```python
from build123d import *

# Parameters (mm, degrees)
SKETCH1_R           = 3.5
BOSS_EXTRUDE1_DEPTH = 10
FILLET1_R           = 2
SKETCH4_R           = 4.5
CUT_EXTRUDE1_DEPTH  = 26
FILLET2_R           = 2


with BuildPart() as part:
    # Sketch1 → Boss-Extrude1 (new body)
    with BuildSketch(Plane.XY):
        with BuildLine():
            Line((57.741071939, 36.562090071), (56.204690111, 51.925908355))
            Line((56.204690111, 51.925908355), (46.264731801, 53.020087861))
            ThreePointArc((46.264731801, 53.020087861), (47.519621722, 46.969136515), (52.091231644, 42.811114916))
            Line((52.091231644, 42.811114916), (52.765885988, 36.064571476))
            Line((52.765885988, 36.064571476), (-12.906568566, 29.49732602))
            Line((-12.906568566, 29.49732602), (-12.011035094, 20.541991308))
            Line((-12.011035094, 20.541991308), (58.63660541, 27.606755359))
            Line((58.63660541, 27.606755359), (67.591940122, 28.50228883))
            Line((67.591940122, 28.50228883), (66.696406651, 37.457623542))
            Line((66.696406651, 37.457623542), (57.741071939, 36.562090071))
        make_face()
        with Locations((58.188838675, 32.084422715)):
            Circle(SKETCH1_R, mode=Mode.SUBTRACT)
    extrude(amount=BOSS_EXTRUDE1_DEPTH)

    # Fillet1
    fillet1_edges = [part.edges().sort_by_distance(p)[0] for p in [
        (56.204690111, 51.925908355, 5),
        (57.741071939, 36.562090071, 5),
        (66.696406651, 37.457623542, 5),
        (67.591940122, 28.50228883, 5),
        (52.765885988, 36.064571476, 5),
    ]]
    fillet(fillet1_edges, radius=FILLET1_R)

    # Sketch4 → Cut-Extrude1 (cut)
    with BuildSketch(Plane(origin=(0, 0, 0), x_dir=(1, 0, 0), z_dir=(0, 1, 0))):
        with Locations(Location((4.295066604, -5, 0), (0, 0, 180))):
            Circle(SKETCH4_R)
    extrude(amount=CUT_EXTRUDE1_DEPTH, mode=Mode.SUBTRACT)

    # Fillet2
    fillet2_edges = [part.edges().sort_by_distance(p)[0] for p in [
        (-12.011035094, 20.541991308, 5),
        (-12.906568566, 29.49732602, 5),
    ]]
    fillet(fillet2_edges, radius=FILLET2_R)


solid = part.part
```
Model file for the job. Use its own axes, mm. A direction names the side the tool comes from. Coordinates: 2 decimals unless noted, no trailing zeros. Order: outer loops, then holes, each group sorted by start corner. A loop starts at its lowest first (then second) coordinate and runs counter-clockwise, first axis right, second up. Notation, with made-up numbers: (-9.5, 46) -> (16.5, 46) arc R29 cw to (16.5, 72) -> close; hole circle Ø10 at (-12, 29). An arc over 180 degrees is marked (long way). Answer as a JSON object with one key per item and string values. Group by question number.
1) Which spindle directions (+Z, -Z, +X, -X, +Y, -Y) get a long thin tool onto all of the face, cutting with end or side? Do faces 1 (the face through (52.326, 40.466, 4.93)), 2 (the face through (62.254, 37.013, 4.93)), 3 (the face through (56.962, 44.351, 4.93)), 4 (the face through (4, 26, 5)). Say none if no direction does.
2) Flat gauge pins, fed straight in: pin 1 (4.5 mm diameter, centred on x = 6, z = 6, fed in from -Y); pin 2 (3 mm diameter, centred on x = 35, z = 4, fed in from -Y); pin 3 (2 mm diameter, centred on x = 32, y = 24, fed in from -Z); pin 4 (4 mm diameter, centred on y = 42.5, z = 7, fed in from +X). Where does each tip first touch, or does it go through?
3) Cut at B-B, the plane x = 48. Write the cut outline in (y, z).
4) Pull direction Z, two halves, no side cores. Call faces 5 (the face through (52.14, 36.61, 5.07)), 6 (the face through (30, 30, 10)), 7 (the face through (0.138, 24.307, 3.276)): +Z half, -Z half, draft (parallel to the pull), parting line (faces both ways), or undercut.
5) Drill centre lines: L1, parallel to Z at x = 3, y = 23; L2, parallel to Y at x = 8.5, z = 2.5; L3, parallel to X at y = 29, z = 4.5. Where is each one in solid material? Low to high.
6) Cut at A-A, the plane z = 6.5. Write the cut outline in (x, y).
7) Cut at D-D, the plane y = 46.5. Write the cut outline in (x, z), then the cut area to 3 significant figures.
8) Cut at C-C, the plane z = 1.25. Write the cut outline in (x, y).
Check values:
{
 "1": {"face 1": "+Z, -Z, -X", "face 2": "+Z, -Z, +Y", "face 3": "+Z, -Z, +X, +Y", "face 4": "-Y"},
 "2": {"pin 1": "stops at y = 26", "pin 2": "stops at y = 25.09", "pin 3": "stops at z = 0", "pin 4": "stops at x = 57.35"},
 "3": {"outline": "(26.54, 0) -> (35.59, 0) -> (35.59, 10) -> (26.54, 10) -> close; (46.21, 0) -> (52.83, 0) -> (52.83, 10) -> (46.21, 10) -> close"},
 "4": {"face 5": "draft", "face 6": "+Z half", "face 7": "undercut"},
 "5": {"L1": "z = 0 to 0.69, 9.31 to 10", "L2": "y = 22.59 to 31.64", "L3": "x = -12.24 to 56.53, 59.84 to 66.93"},
 "6": {"outline": "(-12.71, 27.51) -> (-12.21, 22.53) arc R2 ccw to (-10.02, 20.74) -> (0.05, 21.75) -> (0.05, 26) -> (8.54, 26) -> (8.54, 22.6) -> (65.6, 28.3) arc R2 ccw to (67.39, 30.49) -> (66.9, 35.47) arc R2 ccw to (64.71, 37.26) -> (59.73, 36.76) arc R2 cw to (57.54, 38.55) -> (56.37, 50.31) arc R2 ccw to (54.59, 52.1) -> (46.26, 53.02) arc R10 ccw to (52.09, 42.81) -> (52.57, 38.05) arc R2 cw to (50.78, 35.87) -> (-10.92, 29.7) arc R2 ccw to start; hole circle Ø7 at (58.19, 32.08)"},
 "7": {"outline": "(47.8, 0) -> (56.75, 0) -> (56.75, 10) -> (47.8, 10) -> close", "area": "89.4 mm²"},
 "8": {"outline": "(-12.71, 27.51) -> (-12.21, 22.53) arc R2 ccw to (-10.02, 20.74) -> (1.81, 21.92) -> (1.81, 26) -> (6.78, 26) -> (6.78, 22.42) -> (65.6, 28.3) arc R2 ccw to (67.39, 30.49) -> (66.9, 35.47) arc R2 ccw to (64.71, 37.26) -> (59.73, 36.76) arc R2 cw to (57.54, 38.55) -> (56.37, 50.31) arc R2 ccw to (54.59, 52.1) -> (46.26, 53.02) arc R10 ccw to (52.09, 42.81) -> (52.57, 38.05) arc R2 cw to (50.78, 35.87) -> (-10.92, 29.7) arc R2 ccw to start; hole circle Ø7 at (58.19, 32.08)"}
}
